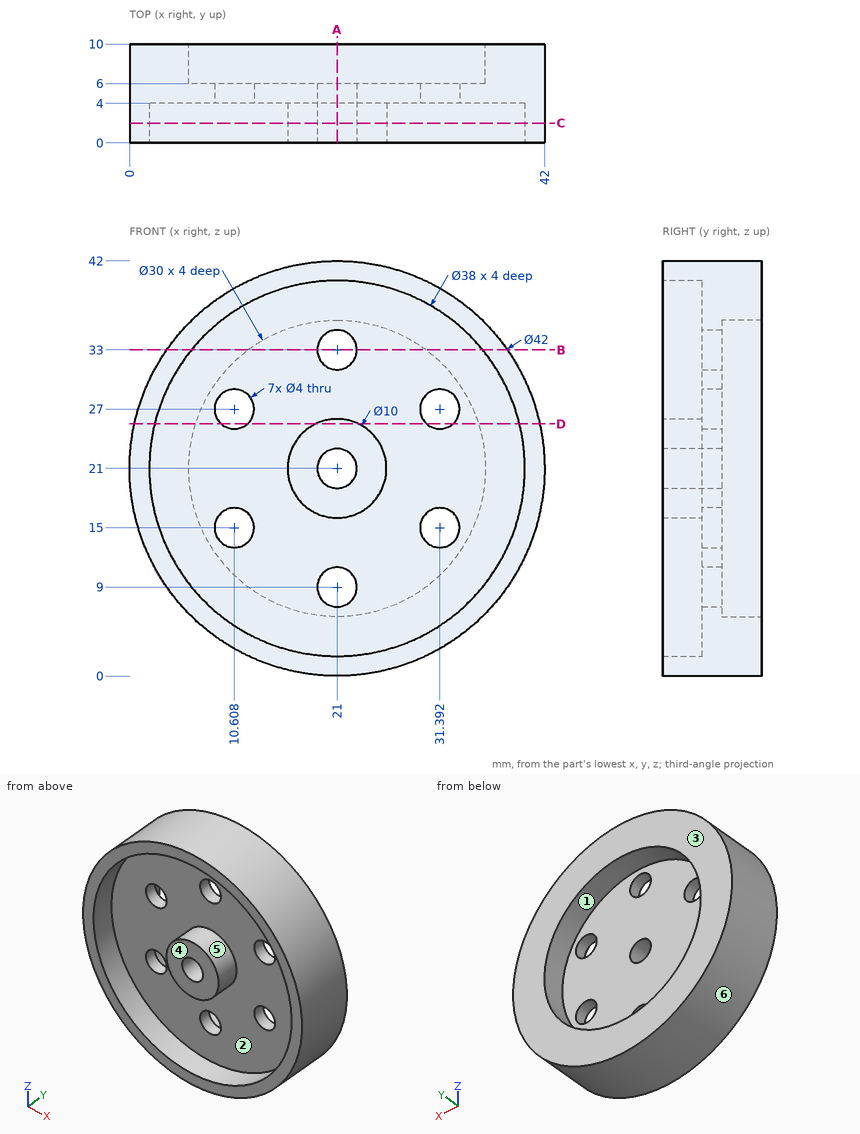
Input: dimensioned drawing with shaded views. Units: mm. Origin: part minimum x, y, z. A direction names the side the tool comes from. Round coordinates to 2 decimals unless told otherwise and drop trailing zeros. Order: outer loops, then holes, each group sorted by start corner. A loop starts at its lowest first (then second) coordinate and runs counter-clockwise, first axis right, second up. Notation, with made-up numbers: (78.25, 6) - (107.25, 6) arc R19 cw to (107.25, 21) - close; hole circle Ø1 at (55, 88.25). An arc over 180 degrees is marked (long way). Answer as a JSON object with one key per item and string values. Group by question number.
(1) Reachability of the marked faces 1, 2 and 3 from +Z, -Z, +X, -X, +Y, -Y: full face, straight path, thin tool, end or side. Return the list, or none.
(2) Material intervals for probe 1 along Z at (x, y) = (12, 5) (1 decimal); probe 2 along X at (y, z) = (9.15, 21); probe 3 along Z at (x, y) = (25.5, 3.75) (1 decimal), sorted ascending. Write a range as from..to.
(3) Cut plane B-B (z = 33). Return loops of the section in (x, y).
(4) Cut plane C-C (y = 2). Return loops of the section in (x, z).
(5) Cut plane A-A (x = 21). Return loops of the section in (y, z).
(6) Cut plane D-D (z = 25.5). Return loops of the section in (x, y) (1 decimal), then the cut area to 3 significant figures.
(7) Pin query (flat end, axial travel): P1, Ø5, axis at y = 6, z = 13, coming from the +X side; P2, Ø9, axis at x = 13.5, z = 14, coming from the +Y side; P3, Ø1.5, axis at y = 4.5, z = 23, coming from the -X side; P4, Ø5, axis at x = 21, z = 21, coming from the -Y side. Return the tip coordinate at first contact, or that it passes through.
(8) Draft query along Z for the marked faces 4, 5 and 6. Return one class per face: released by +Z, released by -Z, zero draft, split by the parting line, or undercut.
Here are the results:
{
 "1": {"face 1": "+Y", "face 2": "-Y", "face 3": "+Z, -Z, +X, -X, +Y"},
 "2": {"probe 1": "z = 2..13.6, 16.4..25.6, 28.4..40", "probe 2": "x = 0..6, 36..42", "probe 3": "z = 0.5..2.5, 18.8..23.2, 39.5..41.5"},
 "3": {"outline": "(3.77, 0) - (6.27, 0) - (6.27, 4) - (19, 4) - (19, 6) - (12, 6) - (12, 10) - (3.77, 10) - close; (23, 4) - (35.73, 4) - (35.73, 0) - (38.23, 0) - (38.23, 10) - (30, 10) - (30, 6) - (23, 6) - close"},
 "4": {"outline": "circle Ø42 at (21, 21); circle Ø10 at (21, 21); hole circle Ø38 at (21, 21); hole circle Ø4 at (21, 21)"},
 "5": {"outline": "(0, 0) - (10, 0) - (10, 6) - (6, 6) - (6, 7) - (4, 7) - (4, 2) - (0, 2) - close; (0, 16) - (4, 16) - (4, 11) - (6, 11) - (6, 19) - (0, 19) - close; (0, 23) - (6, 23) - (6, 31) - (4, 31) - (4, 26) - (0, 26) - close; (0, 40) - (4, 40) - (4, 35) - (6, 35) - (6, 36) - (10, 36) - (10, 42) - (0, 42) - close"},
 "6": {"outline": "(0.5, 0) - (2.5, 0) - (2.5, 4) - (9.3, 4) - (9.3, 6) - (6.7, 6) - (6.7, 10) - (0.5, 10) - close; (11.9, 4) - (18.8, 4) - (18.8, 0) - (23.2, 0) - (23.2, 4) - (30.1, 4) - (30.1, 6) - (11.9, 6) - close; (32.7, 4) - (39.5, 4) - (39.5, 0) - (41.5, 0) - (41.5, 10) - (35.3, 10) - (35.3, 6) - (32.7, 6) - close", "area": "155 mm^2"},
 "7": {"P1": "stops at x = 41.27", "P2": "stops at y = 6", "P3": "stops at x = 0.04", "P4": "stops at y = 0"},
 "8": {"face 4": "zero draft", "face 5": "undercut", "face 6": "split by the parting line"}
}
